from build123d import *

# Parameters (mm, degrees)
F1_DEPTH = 2.54
F2_R     = 2.159
F3_R     = 2.7051
F4_R     = 2.54
F5_DEPTH = 2.54


with BuildPart() as f1:
    # F0 (on Top) → F1 (new body)
    with BuildSketch(Plane.XY):
        with BuildLine():
            Line((-9.525, 69.088), (-9.525, 54.8044364171))
            ThreePointArc((-9.525, 54.8044364171), (-48.1735291109, 27.813), (-52.2245341773, -19.1533262375))
            Line((-52.2245341773, -19.1533262375), (-64.5944630967, -26.295108029))
            Line((-64.5944630967, -26.295108029), (-55.0694630967, -42.792891971))
            Line((-55.0694630967, -42.792891971), (-42.6995341773, -35.6511101796))
            ThreePointArc((-42.6995341773, -35.6511101796), (0, -55.626), (42.6995341773, -35.6511101796))
            Line((42.6995341773, -35.6511101796), (55.0694630967, -42.792891971))
            Line((55.0694630967, -42.792891971), (64.5944630967, -26.295108029))
            Line((64.5944630967, -26.295108029), (52.2245341773, -19.1533262375))
            ThreePointArc((52.2245341773, -19.1533262375), (48.1735291109, 27.813), (9.525, 54.8044364171))
            Line((9.525, 54.8044364171), (9.525, 69.088))
            Line((9.525, 69.088), (-9.525, 69.088))
        make_face()
        with BuildLine():
            ThreePointArc((0, 13.462), (9.5190714883, 9.5190714883), (13.462, 0))
            ThreePointArc((13.462, 0), (-9.5190714883, -9.5190714883), (0, 13.462))
        make_face(mode=Mode.SUBTRACT)
    extrude(amount=F1_DEPTH)

    # F2 (on Top) + F3 (on Top) + F4 (on Top) → F5 (cut)
    with BuildSketch(Plane.XY):
        with Locations((0, 19.05)):
            Circle(F2_R)
        with Locations((0, -19.05)):
            Circle(F2_R)
    with BuildSketch(Plane.XY):
        with Locations((0, 55.519441794)):
            Circle(F3_R)
        with Locations((-48.1168723708, -27.697924297)):
            Circle(F3_R)
        with Locations((48.0812469975, -27.759720897)):
            Circle(F3_R)
    with BuildSketch(Plane.XY):
        with Locations((-41.9043712129, 24.1935)):
            Circle(F4_R)
        with Locations((41.9043712129, 24.1935)):
            Circle(F4_R)
        with Locations((0, -48.387)):
            Circle(F4_R)
    extrude(amount=F5_DEPTH, mode=Mode.SUBTRACT)


solid = f1.part
Check sheet for the modelled part. Datum: model origin and axes. Units: mm. A direction names the side the tool comes from. Give positions to 0.01 mm unless a question says otherwise; leave off trailing zeros. Write each loop counter-clockwise with the first axis right and the second up, starting at its lowest first coordinate (ties: lowest second). Pieces come first, ordered by that corner, then holes. Notation, with made-up numbers: (-33, -23.75) -> (-14, -23.75) arc R15 cw to (-14, 1.25) -> close; hole circle Ø2 at (-8, 87). An arc over 180 degrees is marked (long way). Use one line per item in the form item = value. Start each with the question number.
1. Section check B-B (y = -2). Record the cut outline in (x, z).
2. Section check D-D (x = 23.5). Record the cut outline in (y, z).
3. Access from +Z, -Z, +X, -X, +Y, -Y to the whole of each face (thin tool, end or side, straight path). Record for faces 5 (the cylindrical face through (-0.468, -21.158, 1.252)), 6 (the flat face through (48.798, -39.172, 1.252)), 7 (the flat face through (-58.323, -22.674, 1.252)).
4. Section check A-A (y = -40). Record the cut outline in (x, z), and give its area (3 significant figures).
5. Section check C-C (z = 0.6). Count the separate pieces of the cut face and the enclosed holes in it, and give its area (3 significant figures).
6. Mould release check, pull along Y, two halves, no side actions. Record for faces 1 (the flat face through (13, -6, 2.54)), 2 (the cylindrical face through (40.03, 25.91, 1.25)), 3 (the cylindrical face through (48.51, 27.22, 1.25)), 4 (the flat face through (59.765, -34.659, 1.252)): pulls with the +Y half, pulls with the -Y half, needs draft (parallel to the pull), parting line crosses it, or undercut.
7. Thickness scan on line 1 along Y through (x, z) = (0, 1.55); line 2 along X through (y, z) = (-28, 0.6); line 3 along X through (y, z) = (10.5, 0.6). Record the ranges inside material, lowest first. Write a range as from..to.
8. Go/stop test with flat-tipped pins: P1, Ø8, axis at x = -37, y = 42.5, coming from the -Z side; P2, Ø1.5, axis at y = 10, z = 2, coming from the +X side. Record where each tip stops, or that it passes through.
Conclusion:
q1.outline = (-55.59, 0) -> (-13.31, 0) -> (-13.31, 2.54) -> (-55.59, 2.54) -> close; (13.31, 0) -> (55.59, 0) -> (55.59, 2.54) -> (13.31, 2.54) -> close
q2.outline = (-50.42, 0) -> (50.42, 0) -> (50.42, 2.54) -> (-50.42, 2.54) -> close
q3.face_5 = +Z, -Z
q3.face_6 = +Z, -Z, -Y
q3.face_7 = +Z, -Z, -X
q4.outline = (-56.68, 0) -> (-50.23, 0) -> (-50.23, 2.54) -> (-56.68, 2.54) -> close; (-38.66, 0) -> (38.66, 0) -> (38.66, 2.54) -> (-38.66, 2.54) -> close; (50.23, 0) -> (56.68, 0) -> (56.68, 2.54) -> (50.23, 2.54) -> close
q4.area = 229 mm²
q5.separate_pieces = 1
q5.enclosed_holes = 9
q5.area = 9,780 mm²
q6.face_1 = needs draft
q6.face_2 = undercut
q6.face_3 = undercut
q6.face_4 = pulls with the -Y half
q7.line_1 = -55.63..-50.93, -45.85..-21.21, -16.89..-13.46, 13.46..16.89, 21.21..52.81, 58.22..69.09
q7.line_2 = -63.61..-50.81, -45.43..45.39, 50.78..63.61
q7.line_3 = -54.63..-8.42, 8.42..54.63
q8.P1 = 0
q8.P2 = 54.85
